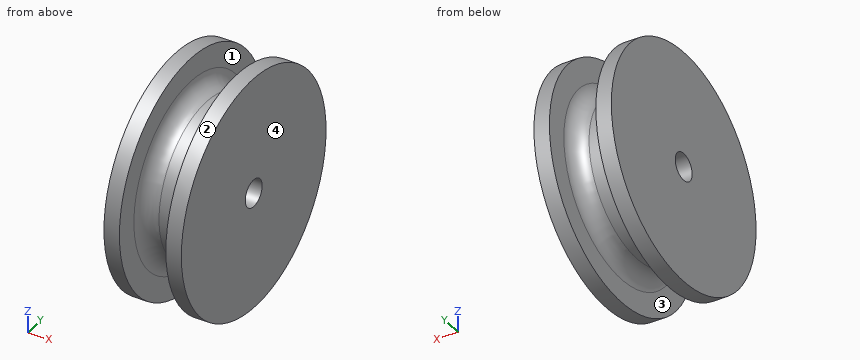
```python
from build123d import *


with BuildPart() as part:
    # Sketch1 → Revolve1 (revolve)
    with BuildSketch(Plane.XY):
        with BuildLine():
            Line((-1, 10), (1, 10))
            ThreePointArc((1, 10), (2.414213562, 10.585786438), (3, 12))
            Line((3, 12), (3, 15))
            Line((3, 15), (5, 15))
            Line((5, 15), (5, 1.753554502))
            Line((5, 1.753554502), (-5, 1.753554502))
            Line((-5, 1.753554502), (-5, 15))
            Line((-5, 15), (-3, 15))
            Line((-3, 15), (-3, 12))
            ThreePointArc((-3, 12), (-2.414213562, 10.585786438), (-1, 10))
        make_face()
    revolve(axis=Axis((-9.241706161, 0, 0), (1, 0, 0)))


solid = part.part
```
For this review, take the finished solid that the model builds, in its own axes (mm). Face numbers are marked on the shaded views. Round coordinates to 2 decimals unless told otherwise and drop trailing zeros. Write each loop counter-clockwise with the first axis right and the second up, starting at its lowest first coordinate (ties: lowest second). Pieces come first, ordered by that corner, then holes. Notation, with made-up numbers: (39, 4) -> (86, 4) arc R22 cw to (86, 37) -> close; hole circle Ø8 at (-33, 75.25). An arc over 180 degrees is marked (long way). Use one line per item in the form item = value.
1) To check wall thickness, follow L1, parallel to Z at x = 1, y = 0; L2, parallel to X at y = 10.5, z = 10; L3, parallel to X at y = -8.75, z = 6.5. State the ranges of each line that lie inside material, in increasing order. Write a range as from..to.
Found:
L1 = -10..-1.75, 1.75..10
L2 = -5..-3, 3..5
L3 = -5..-2.67, 2.67..5
2) Take a section at C-C, the plane x = -3.5. Write out the cut boundary in (y, z), and give its area (3 significant figures).
Found:
outline = circle Ø30 at (0, 0); hole circle Ø3.51 at (0, 0)
area = 697 mm2
3) Mouldability with a two-part tool opening along X and no side actions: class the marked faces 1, 2, 3 and 4 as +X half, -X half, draft (parallel to the pull), parting line (faces both ways), or undercut.
Found:
face_1 = undercut
face_2 = draft
face_3 = undercut
face_4 = +X half
4) Take a section at D-D, the plane x = 2. Write out the cut boundary in (y, z), and give its area (3 significant figures).
Found:
outline = circle Ø20.54 at (0, 0); hole circle Ø3.51 at (0, 0)
area = 322 mm2
5) Take a section at A-A, the plane z = 0. Write out the cut boundary in (x, y).
Found:
outline = (-5, -15) -> (-3, -15) -> (-3, -12) arc R2 cw to (-1, -10) -> (1, -10) arc R2 cw to (3, -12) -> (3, -15) -> (5, -15) -> (5, -1.75) -> (-5, -1.75) -> close; (-5, 1.75) -> (5, 1.75) -> (5, 15) -> (3, 15) -> (3, 12) arc R2 cw to (1, 10) -> (-1, 10) arc R2 cw to (-3, 12) -> (-3, 15) -> (-5, 15) -> close
6) Clearance check with a flat-ended pin moving along its axis: pin 1 (1.5 mm diameter, centred on x = 4, z = 10, fed in from +Y). State where the tip first meets the part, or that it passes through.
Found:
pin_1 = 11.81
